Design review of the part built by this model. Coordinates are the model's own, in mm. Give positions to 0.01 mm unless a question says otherwise; leave off trailing zeros. Write each loop counter-clockwise with the first axis right and the second up, starting at its lowest first coordinate (ties: lowest second). Pieces come first, ordered by that corner, then holes. Notation, with made-up numbers: M -14.5,-27.5 L 12.5,-27.5 A22 ccw 12.5,-14.5 Z; hole C 29,20.25 d10. An arc over 180 degrees is marked long. Use one line per item in the form item = value. Start each with the question number.
from build123d import *

# Parameters (mm, degrees)
F0_W           = 90
F0_H           = 40
F1_DEPTH       = 6.35
F3_D           = 4.2
F4_D           = 6.6
F4_CSINK_D     = 13.44
F4_CSINK_ANGLE = 90


with BuildPart() as f1:
    # F0 (on Top) → F1 (new body)
    with BuildSketch(Plane.XY):
        Rectangle(F0_W, F0_H)
    extrude(amount=F1_DEPTH)

    # F3 (through all)
    with Locations(Plane.XY.offset(6.35)):
        with Locations((-38.99, -1.46), (38.99, -1.46)):
            Hole(F3_D / 2)

    # F4 (through all)
    with Locations(Plane.XY.offset(6.35)):
        with Locations((-25.4, 0), (25.4, 0)):
            CounterSinkHole(F4_D / 2, F4_CSINK_D / 2, counter_sink_angle=F4_CSINK_ANGLE)


solid = f1.part
1. Clearance check with flat-ended pins moving along their axes: pin 1 Ø2.5 at (x, y) = (-38.99, -1.46) entering from +Z; pin 2 Ø10.5 at (x, y) = (-25.4, 0) entering from +Z. State where each tip first meets the part, or that it passes through.
2. Draft analysis for pull direction Y (two halves, no side actions). For faces 1 (the conical face through (28.863, 0.152, 3.096)), 2 (the flat face through (-1, 0, 6.35)), 3 (the cylindrical face through (22.35, -1.26, 1.44)), 4 (the flat face through (-1, 20, 3)), state which applies: pulls with the +Y half, pulls with the -Y half, needs draft (parallel to the pull), parting line crosses it, or undercut.
3. We need section B-B (z = 5). State the section outline as (x, y) points.
4. We need section A-A (x = -38.99). State the section outline as (y, z) points, and give its area (3 significant figures).
5. We need section C-C (x = 25.4). State the section outline as (y, z) points.
6. To check wall thickness, follow L1, parallel to Y at x = 25.4, z = 1.35; L2, parallel to X at y = 0, z = 2.25; L3, parallel to Y at x = 38.99, z = 1.5. State the ranges of each line that lie inside material, in increasing order.
7. We need section D-D (y = -1.46). Give the number of separate pieces and of enclosed holes in the cut face, and give its area (3 significant figures).
Answer block:
q1.pin_1 = through
q1.pin_2 = 4.88
q2.face_1 = undercut
q2.face_2 = needs draft
q2.face_3 = undercut
q2.face_4 = pulls with the +Y half
q3.outline = M -45,-20 L 45,-20 L 45,20 L -45,20 Z; hole C -38.99,-1.46 d4.2; hole C -25.4,0 d10.74; hole C 25.4,0 d10.74; hole C 38.99,-1.46 d4.2
q4.outline = M -20,0 L -3.56,0 L -3.56,6.35 L -20,6.35 Z; M 0.64,0 L 20,0 L 20,6.35 L 0.64,6.35 Z
q4.area = 227 mm^2
q5.outline = M -20,0 L -3.3,0 L -3.3,2.93 L -6.72,6.35 L -20,6.35 Z; M 3.3,0 L 20,0 L 20,6.35 L 6.72,6.35 L 3.3,2.93 Z
q6.L1 = -20 to -3.3, 3.3 to 20
q6.L2 = -45 to -40.5, -37.48 to -28.7, -22.1 to 22.1, 28.7 to 37.48, 40.5 to 45
q6.L3 = -20 to -3.56, 0.64 to 20
q7.separate_pieces = 5
q7.enclosed_holes = 0
q7.area = 418 mm^2
